from build123d import *

# Parameters (mm, degrees)
BOSS_EXTRUDE1_DEPTH = 1.6
SKETCH2_W           = 16.5
SKETCH2_H           = 16.5
BOSS_EXTRUDE2_DEPTH = 2
BOSS_EXTRUDE3_DEPTH = 4.4
SKETCH5_W           = 4
SKETCH5_H           = 10.5
BOSS_EXTRUDE4_DEPTH = 4.4
SKETCH6_W           = 9
SKETCH6_H           = 4
BOSS_EXTRUDE5_DEPTH = 2.5


with BuildPart() as part:
    # Sketch1 → Boss-Extrude1 (new body)
    with BuildSketch(Plane(origin=(0, 0, 0), x_dir=(0, 1, 0), z_dir=(0, 0, 1))):
        with BuildLine():
            Line((-8, 10), (8, 10))
            ThreePointArc((8, 10), (9.414213562, 9.414213562), (10, 8))
            Line((10, 8), (10, -8))
            ThreePointArc((10, -8), (9.414213562, -9.414213562), (8, -10))
            Line((8, -10), (-8, -10))
            ThreePointArc((-8, -10), (-9.414213562, -9.414213562), (-10, -8))
            Line((-10, -8), (-10, 8))
            ThreePointArc((-10, 8), (-9.414213562, 9.414213562), (-8, 10))
        make_face()
    extrude(amount=BOSS_EXTRUDE1_DEPTH)

    # Sketch2 → Boss-Extrude2 (add)
    with BuildSketch(Plane.XY.offset(1.6)):
        Rectangle(SKETCH2_W, SKETCH2_H)
    extrude(amount=BOSS_EXTRUDE2_DEPTH)

    # Sketch3 → Boss-Extrude3 (add)
    with BuildSketch(Plane.XY.offset(3.6)):
        with BuildLine():
            Line((6.5, 7.5), (7.5, 6.5))
            Line((7.5, 6.5), (7.5, -6.5))
            ThreePointArc((7.5, -6.5), (7.207106781, -7.207106781), (6.5, -7.5))
            Line((6.5, -7.5), (-6.5, -7.5))
            ThreePointArc((-6.5, -7.5), (-7.207106781, -7.207106781), (-7.5, -6.5))
            Line((-7.5, -6.5), (-7.5, 6.5))
            ThreePointArc((-7.5, 6.5), (-7.207106781, 7.207106781), (-6.5, 7.5))
            Line((-6.5, 7.5), (6.5, 7.5))
        make_face()
    extrude(amount=BOSS_EXTRUDE3_DEPTH)

    # Sketch5 → Boss-Extrude4 (add)
    with BuildSketch(Plane(origin=(0, 0, 0), x_dir=(1, 0, 0), z_dir=(0, 0, -1))):
        with Locations((-8, 0)):
            Rectangle(SKETCH5_W, SKETCH5_H)
        with Locations((8, 0)):
            Rectangle(SKETCH5_W, SKETCH5_H)
    extrude(amount=BOSS_EXTRUDE4_DEPTH)

    # Sketch6 → Boss-Extrude5 (add)
    with BuildSketch(Plane(origin=(10, 0, 0), x_dir=(0, -1, 0), z_dir=(-1, 0, 0))):
        with Locations((0, -2)):
            Rectangle(SKETCH6_W, SKETCH6_H)
    extrude(amount=-BOSS_EXTRUDE5_DEPTH)


solid = part.part
Input: part model. Units: mm. Frame: model coordinates. A direction names the side the tool comes from. Give positions to 0.01 mm unless a question says otherwise; leave off trailing zeros. Loops run counter-clockwise (first coordinate to the right, second up) from the corner with the lowest first, then second, coordinate; pieces in that order, holes last. Notation, with made-up numbers: M 72.5,18 L 117.5,18 A20 ccw 117.5,56 Z; hole C 71.25,74.25 d3. An arc over 180 degrees is marked long. Use CSV: the item, a comma, the result in double quotes.
(1) Set-up query: faces 5 (the face through (11, 4.5, -2)), 6 (the face through (7.215, -7.199, 5.769)), 7 (the face through (8, 0, 3.6)). Return all of +Z, -Z, +X, -X, +Y, -Y with unobstructed straight access to the full face (end or side cutting, diameter ignored); none if empty.
Outcome:
face 5,"+Z, -Z, +X, +Y"
face 6,"+Z, +X, -Y"
face 7,"+Z"
(2) Pin query (flat end, axial travel): P1, Ø2, axis at x = -8.5, z = -2.5, coming from the -Y side; P2, Ø2, axis at y = 1.5, z = 6.5, coming from the +X side; P3, Ø2, axis at x = 8, z = -3, coming from the +Y side. Return the tip coordinate at first contact, or that it passes through.
Outcome:
P1,"stops at y = -5.25"
P2,"stops at x = 7.5"
P3,"stops at y = 5.25"
(3) Section B-B, the plane y = 5.75. Return loops of the section in (x, z).
Outcome:
outline,"M -10,0 L 10,0 L 10,1.6 L 8.25,1.6 L 8.25,3.6 L 7.5,3.6 L 7.5,8 L -7.5,8 L -7.5,3.6 L -8.25,3.6 L -8.25,1.6 L -10,1.6 Z"
(4) Section A-A, the plane z = -3.5. Return loops of the section in (x, y).
Outcome:
outline,"M -10,-5.25 L -6,-5.25 L -6,5.25 L -10,5.25 Z; M 6,-5.25 L 10,-5.25 L 10,-4.5 L 12.5,-4.5 L 12.5,4.5 L 10,4.5 L 10,5.25 L 6,5.25 Z"
(5) Pull-direction query (X, two-part tool) for faces 1 (the face through (6, 0, -2)), 2 (the face through (0, 0, 0)), 3 (the face through (-7.215, 7.199, 5.769)), 4 (the face through (11, -4.5, -2)); classes: pulls with the +X half, pulls with the -X half, needs draft (parallel to the pull), parting line crosses it, or undercut.
Outcome:
face 1,"undercut"
face 2,"undercut"
face 3,"pulls with the -X half"
face 4,"needs draft"
(6) Material intervals for L1, parallel to X at y = 1.75, z = -2.5; L2, parallel to Z at x = -1.75, y = -6.5; L3, parallel to Y at x = -1.25, z = 5.5, sorted ascending. Write a range as [from, to].
Outcome:
L1,"x = [-10, -6], [6, 12.5]"
L2,"z = [0, 8]"
L3,"y = [-7.5, 7.5]"
(7) Section D-D, the plane z = 6.5. Return loops of the section in (x, y), plus the area to 3 significant figures.
Outcome:
outline,"M -7.5,-6.5 A1 ccw -6.5,-7.5 L 6.5,-7.5 A1 ccw 7.5,-6.5 L 7.5,6.5 L 6.5,7.5 L -6.5,7.5 A1 ccw -7.5,6.5 Z"
area,"224 mm²"
